Check sheet for the drawn part. Datum: minimum x, y, z corner. Units: mm. Give positions to 0.01 mm unless a question says otherwise; leave off trailing zeros. Write each loop counter-clockwise with the first axis right and the second up, starting at its lowest first coordinate (ties: lowest second). Pieces come first, ordered by that corner, then holes. Notation, with made-up numbers: (58, -1.5) - (104, -1.5) arc R28 cw to (104, 30.5) - close; hole circle Ø10 at (23.5, 41). An arc over 180 degrees is marked (long way). Answer as a JSON object with one key per item and string values. Group by question number.
Item 1: Sectioned sample at A-A, the plane z = 6.5. Record the boundary of the cut face in (x, y), and give its area (3 significant figures).
Item 2: Go/stop test with a flat-tipped pin: pin 1 (3 mm diameter, centred on x = 35.5, y = 13, fed in from -Z). Record where the tip stops, or that it passes through.
Item 3: Scan lines: line 1 along X through (y, z) = (10.25, 8.5); line 2 along X through (y, z) = (6, 6). Record each from-to range of solid material in increasing order. Write a range as [from, to].
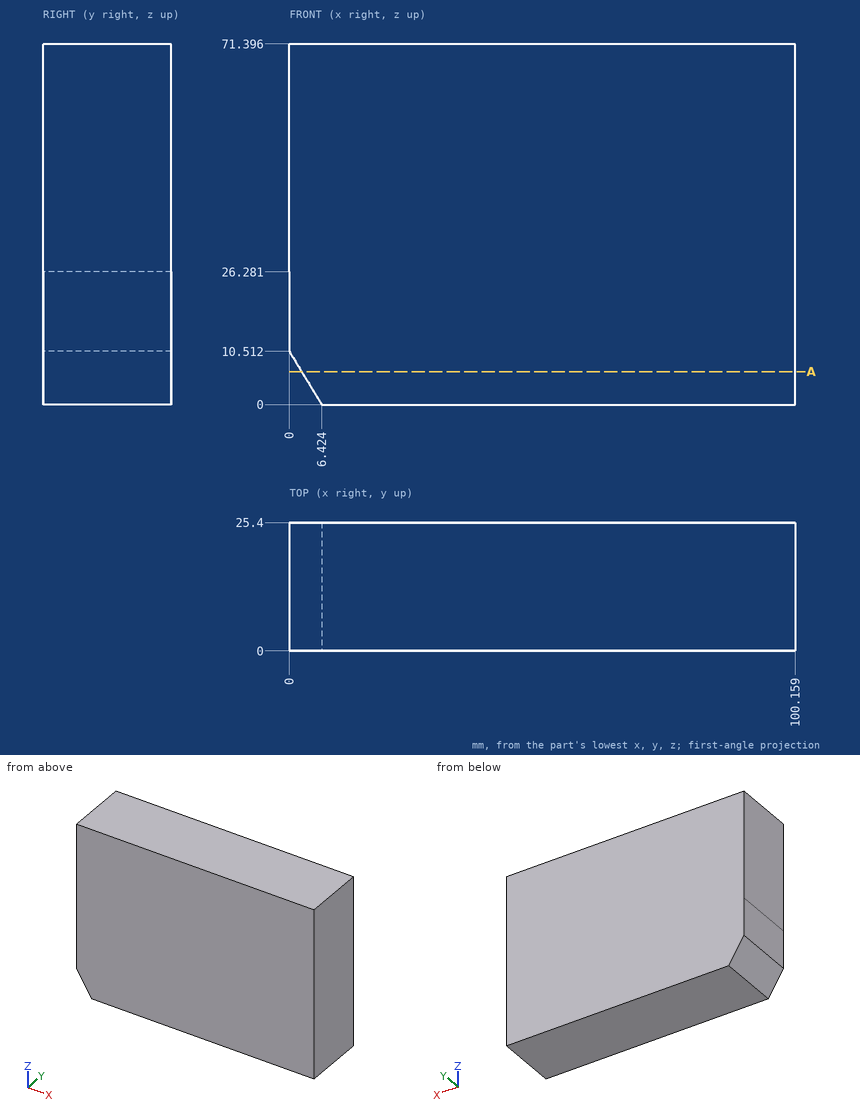
Geometry check:
{
 "1": {"outline": "(2.45, 0) - (100.16, 0) - (100.16, 25.4) - (2.45, 25.4) - close", "area": "2,480 mm^2"},
 "2": {"pin 1": "z = 0"},
 "3": {"line 1": "[1.23, 100.16]", "line 2": "[2.76, 100.16]"}
}
